from build123d import *

# Parameters (mm, degrees)
SKIZZE1_W                       = 135
SKIZZE1_H                       = 80
AUFSATZ_LINEAR_AUSTRAGEN1_DEPTH = 30
SCHALE1_T                       = -2
SKIZZE2_R                       = 6
SCHNITT_LINEAR_AUSTRAGEN1_DEPTH = 30


with BuildPart() as part:
    # Skizze1 → Aufsatz-Linear austragen1 (new body)
    with BuildSketch(Plane(origin=(0, 0, 0), x_dir=(1, 0, 0), z_dir=(0, 1, 0))):
        with Locations((67.5, 40)):
            Rectangle(SKIZZE1_W, SKIZZE1_H)
    extrude(amount=AUFSATZ_LINEAR_AUSTRAGEN1_DEPTH)

    # Schale1
    schale1_openings = [part.faces().sort_by_distance(p)[0] for p in [
        (67.5, 30, -40),
    ]]
    offset(amount=SCHALE1_T, openings=schale1_openings, kind=Kind.INTERSECTION)

    # Skizze2 → Schnitt-Linear austragen1 (cut)
    with BuildSketch(Plane.XY):
        with Locations((20.6, 14.94)):
            Circle(SKIZZE2_R)
        with Locations((34.9, 14.94)):
            Circle(SKIZZE2_R)
        with Locations((49.2, 14.94)):
            Circle(SKIZZE2_R)
        with Locations((63.5, 14.94)):
            Circle(SKIZZE2_R)
        with Locations((77.8, 14.94)):
            Circle(SKIZZE2_R)
    extrude(amount=-SCHNITT_LINEAR_AUSTRAGEN1_DEPTH, mode=Mode.SUBTRACT)


solid = part.part
Model file for the job. Use its own axes, mm. A direction names the side the tool comes from. Coordinates: 2 decimals unless noted, no trailing zeros. Loops run counter-clockwise (first coordinate to the right, second up) from the corner with the lowest first, then second, coordinate; pieces in that order, holes last. Notation, with made-up numbers: (50, 0.5) -> (105, 0.5) arc R20 ccw to (105, 26.5) -> close; hole circle Ø1 at (2.5, 72.25). An arc over 180 degrees is marked (long way). Use one line per item in the form item = value. Start each with the question number.
(1) Pull direction Y, two halves, no side cores. Call faces 1 (the cylindrical face through (77.02, 20.89, -0.99)), 2 (the flat face through (67, 16, -78)), 3 (the cylindrical face through (57.506, 15.204, -0.986)), 4 (the flat face through (67, 0, -41)): pulls with the +Y half, pulls with the -Y half, needs draft (parallel to the pull), parting line crosses it, or undercut.
(2) Cut at D-D on y = 19.25. Give the cut face in (x, z), and give its area (3 significant figures).
(3) Flat gauge pins, fed straight in: pin 1 (3 mm diameter, centred on x = 54.5, y = 25, fed in from +Z); pin 2 (9.5 mm diameter, centred on x = 63.5, y = 14.94, fed in from +Z); pin 3 (1 mm diameter, centred on x = 112, z = -70, fed in from +Y). Where does each tip first touch, or does it go through?
(4) Tool access for faces 5 (the cylindrical face through (54.923, 16.742, -0.986)), 6 (the flat face through (67, 22, -2)), 7 (the flat face through (67, 15, -80)): list every direction of +Z, -Z, +X, -X, +Y, -Y with a clear straight run to the whole face (end or side of a thin tool).
(5) Probe probe 1 along X at (y, z) = (10.75, -20); probe 2 along Y at (x, z) = (49.2, -1.2); probe 3 along Z at (x, y) = (27, 12.5). List the from-to ranges inside material, lowest first. Write a range as from..to.
(6) Cut at B-B on y = 27.25. Give the cut face in (x, z), and give its area (3 significant figures).
(7) Cut at A-A on x = 34.9. Give the cut face in (y, z), and give its area (3 significant figures).
(8) Cut at C-C on z = -12. Give the cut face in (x, y).
Values:
q1.face_1 = undercut
q1.face_2 = needs draft
q1.face_3 = undercut
q1.face_4 = pulls with the -Y half
q2.outline = (0, -80) -> (135, -80) -> (135, 0) -> (81.97, 0) -> (81.97, -2) -> (133, -2) -> (133, -78) -> (2, -78) -> (2, -2) -> (16.43, -2) -> (16.43, 0) -> (0, 0) -> close; (24.77, -2) -> (30.73, -2) -> (30.73, 0) -> (24.77, 0) -> close; (39.07, -2) -> (45.03, -2) -> (45.03, 0) -> (39.07, 0) -> close; (53.37, -2) -> (59.33, -2) -> (59.33, 0) -> (53.37, 0) -> close; (67.67, -2) -> (73.63, -2) -> (73.63, 0) -> (67.67, 0) -> close
q2.area = 761 mm2
q3.pin_1 = 0
q3.pin_2 = -78
q3.pin_3 = 2
q4.face_5 = +Z
q4.face_6 = +Y
q4.face_7 = -Z, +X, -X, +Y, -Y
q5.probe_1 = 0..2, 133..135
q5.probe_2 = 0..8.94, 20.94..30
q5.probe_3 = -80..-78, -2..0
q6.outline = (0, -80) -> (135, -80) -> (135, 0) -> (0, 0) -> close; hole (2, -78) -> (133, -78) -> (133, -2) -> (2, -2) -> close
q6.area = 844 mm2
q7.outline = (0, -80) -> (30, -80) -> (30, -78) -> (2, -78) -> (2, -2) -> (8.94, -2) -> (8.94, 0) -> (0, 0) -> close; (20.94, -2) -> (30, -2) -> (30, 0) -> (20.94, 0) -> close
q7.area = 248 mm2
q8.outline = (0, 0) -> (135, 0) -> (135, 30) -> (133, 30) -> (133, 2) -> (2, 2) -> (2, 30) -> (0, 30) -> close
